Geometry check sheet. Reference: the model listing, model coordinates, mm. Round coordinates to 2 decimals unless told otherwise and drop trailing zeros. Order: outer loops, then holes, each group sorted by start corner. A loop starts at its lowest first (then second) coordinate and runs counter-clockwise, first axis right, second up. Notation, with made-up numbers: (22.5, -26) - (40.5, -26) arc R24 ccw to (40.5, -14) - close; hole circle Ø7 at (63.25, 57). An arc over 180 degrees is marked (long way). Write each question's results on one line, items separated by ' | '.
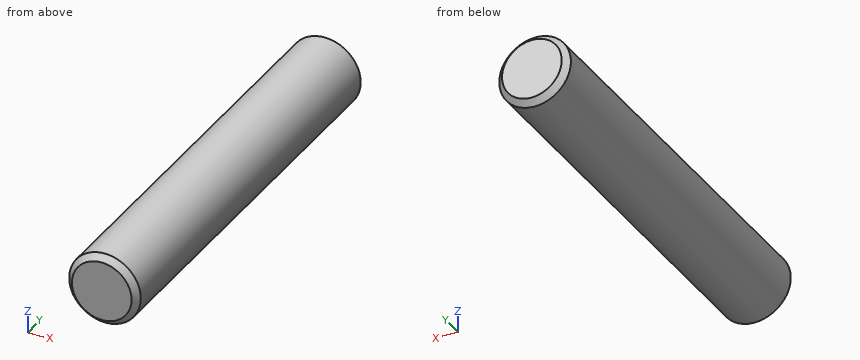
```python
from build123d import *

# Parameters (mm, degrees)
F0_R     = 3
F1_DEPTH = 35
F2_SIZE  = 0.5
F3_SIZE  = 0.5


with BuildPart() as f1:
    # F0 (on Front) → F1 (new body)
    with BuildSketch(Plane.XZ):
        Circle(F0_R)
    extrude(amount=F1_DEPTH)

    # F2
    f2_edges = [f1.edges().sort_by_distance(p)[0] for p in [
        (-3, -35, 0),
    ]]
    chamfer(f2_edges, length=F2_SIZE)

    # F3
    f3_edges = [f1.edges().sort_by_distance(p)[0] for p in [
        (-3, 0, 0),
    ]]
    chamfer(f3_edges, length=F3_SIZE)


solid = f1.part
```
(1) Section check A-A (y = -30). Record the cut outline in (x, z).
Answers follow:
outline: circle Ø6 at (0, 0)
(2) Material ranges on line 1 (X direction, y = -3, z = 0.1); line 2 (X direction, y = -27, z = 1.8), recorded low to high.
Answers follow:
line 1: -3 to 3 | line 2: -2.4 to 2.4
(3) Depth check by flat-ended pin: pin 1 Ø1 at (x, y) = (2.5, -17.5) entering from -Z. Enter the tip coordinate at first touch or a pass-through.
Answers follow:
pin 1: z = -2.24
